Could you check a few things on this drawing? It's one solid part, dimensions in mm from its lowest x, y, z. A direction names the side the tool comes from. Round coordinates to 2 decimals unless told otherwise and drop trailing zeros. Loops run counter-clockwise (first coordinate to the right, second up) from the corner with the lowest first, then second, coordinate; pieces in that order, holes last. Notation, with made-up numbers: (47.5, 60.5) -> (82.5, 60.5) arc R29 ccw to (82.5, 97.5) -> close; hole circle Ø2 at (-34.5, 45). An arc over 180 degrees is marked (long way). Use one line per item in the form item = value. Start each with the question number.
Item 1: If we section it at C-C (z = 33.5): Write out the boundary of the cut face in (x, y).
Item 2: For the marked faces 1 and 2, which set-ups out of +Z, -Z, +X, -X, +Y, -Y let a thin tool reach every point of the face, with its end or its side?
Item 3: If we section it at B-B (z = 8): Write out the boundary of the cut face in (x, y).
Item 4: If we section it at A-A (y = 9.75): Write out the boundary of the cut face in (x, z) (1 decimal), then the cut area to 3 significant figures.
Item 5: If we section it at D-D (y = 4.75): Write out the boundary of the cut face in (x, z), then the cut area to 3 significant figures.
Item 6: Thinking about a two-plate mould opening in X: for the marked faces 3, 4 and 5, which applies, released by +X, released by -X, zero draft, split by the parting line, or undercut?
Item 7: If I drill on L1, parallel to Y at x = 6.75, z = 32.5; L2, parallel to Z at x = 4, y = 7.5; L3, parallel to Y at x = 4.5, z = 35 (1 decimal), over which ranges is the centre line in solid material (lowest first)? Write a range as [from, to].
Item 8: I'm going to push flat-ended pins straight in: pin 1 Ø2.5 at (x, z) = (6.46, 3) entering from +Y; pin 2 Ø8 at (x, z) = (7.5, 28.5) entering from -Y; pin 3 Ø4 at (y, z) = (10.5, 18.5) entering from -X; pin 4 Ø3 at (x, y) = (12, 8.5) entering from -Z. Where does each tip first touch, or does it pass through?
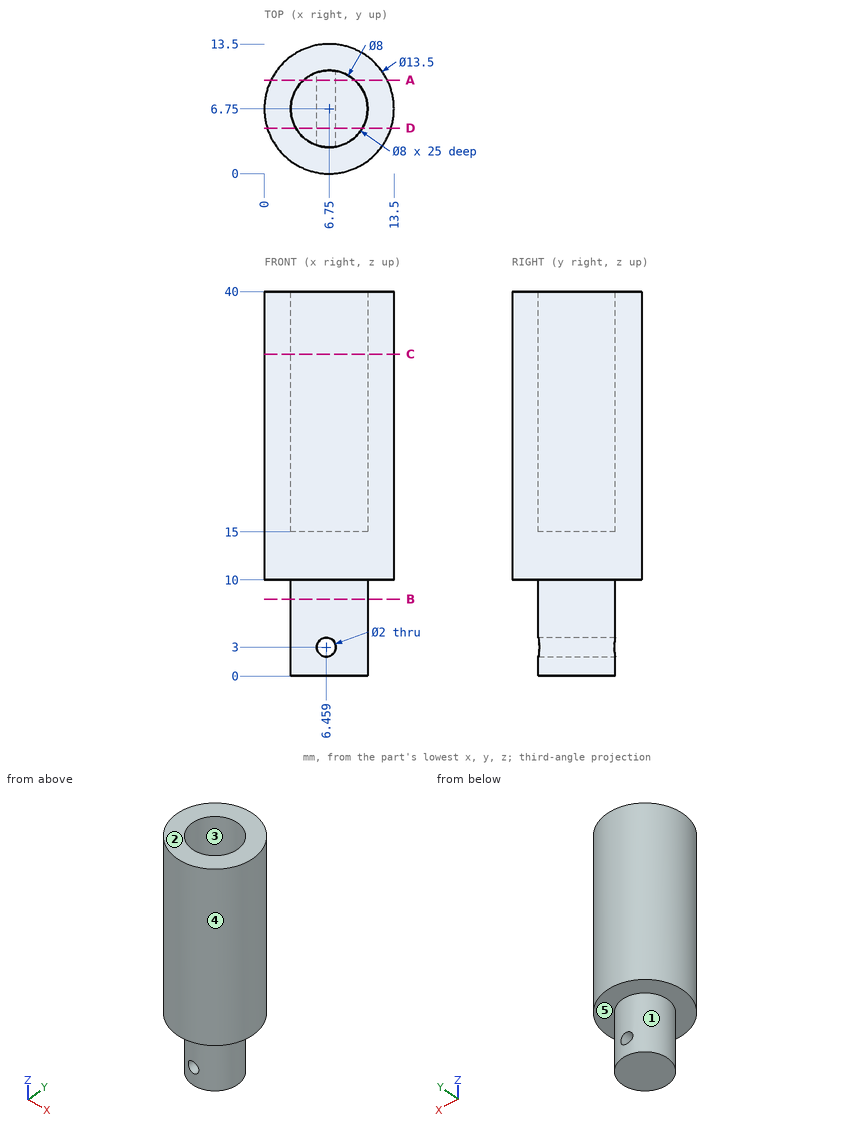
Values found:
q1.outline = circle Ø13.5 at (6.75, 6.75); hole circle Ø8 at (6.75, 6.75)
q2.face_1 = -Z
q2.face_2 = +Z, +X, -X, +Y, -Y
q3.outline = circle Ø8 at (6.75, 6.75)
q4.outline = (0.7, 10) -> (4.1, 10) -> (4.1, 0) -> (9.4, 0) -> (9.4, 10) -> (12.8, 10) -> (12.8, 40) -> (9.4, 40) -> (9.4, 15) -> (4.1, 15) -> (4.1, 40) -> (0.7, 40) -> close; hole circle Ø2 at (6.5, 3)
q4.area = 280 mm2
q5.outline = (0.3, 10) -> (3.29, 10) -> (3.29, 0) -> (10.21, 0) -> (10.21, 10) -> (13.2, 10) -> (13.2, 40) -> (10.21, 40) -> (10.21, 15) -> (3.29, 15) -> (3.29, 40) -> (0.3, 40) -> close; hole circle Ø2 at (6.46, 3)
q5.area = 280 mm2
q6.face_3 = undercut
q6.face_4 = split by the parting line
q6.face_5 = zero draft
q7.L1 = [0, 2.75], [10.75, 13.5]
q7.L2 = [0, 15]
q7.L3 = [0.4, 3.4], [10.1, 13.1]
q8.pin_1 = 10.75
q8.pin_2 = 0
q8.pin_3 = 0.23
q8.pin_4 = 10
